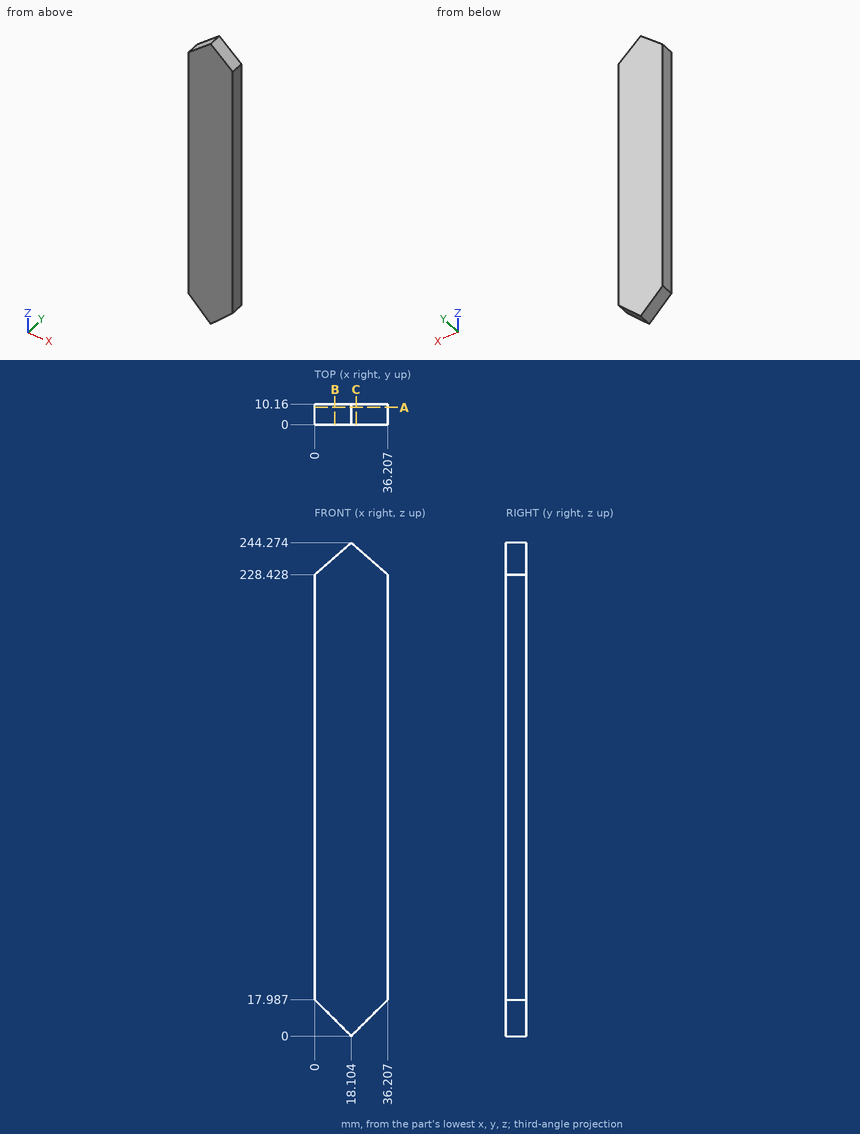
Geometry: see drawing. Coordinates: mm, zero at the bounding-box minimum. Coordinates: 2 decimals unless noted, no trailing zeros. Order: outer loops, then holes, each group sorted by start corner. A loop starts at its lowest first (then second) coordinate and runs counter-clockwise, first axis right, second up. Notation, with made-up numbers: (-18.5, 89.5) -> (-0.5, 89.5) arc R25 ccw to (-0.5, 109.5) -> close; hole circle Ø4 at (-39.75, 67.25). An arc over 180 degrees is marked (long way). Write each question's results on one line, items separated by ' | '. Start each with the question number.
1) Cut plane B-B, the plane x = 10. Output: boundary loops of the cut face in (y, z).
2) Material intervals for line 1 along Z through (x, y) = (14.5, 9); line 2 along Z through (x, y) = (13.5, 4.75) (1 decimal); line 3 along X through (y, z) = (7.5, 231), sorted ascending.
3) First-contact query: pin 1 (4 mm diameter, centred on x = 9.5, y = 7, fed in from +Z) (1 decimal); pin 2 (1.5 mm diameter, centred on x = 7, y = 2.5, fed in from +Z); pin 3 (4 mm diameter, centred on x = 22, y = 6.5, fed in from +Z) (1 decimal). Flat tips, straight axial feed; report the tip coordinate or a pass-through.
4) Cut plane A-A, the plane y = 8.5. Output: boundary loops of the cut face in (x, z), and give its area (3 significant figures).
5) Cut plane C-C, the plane x = 20.5. Output: boundary loops of the cut face in (y, z).
Checks:
1) outline: (0, 8.05) -> (10.16, 8.05) -> (10.16, 237.18) -> (0, 237.18) -> close
2) line 1: 3.58 to 241.12 | line 2: 4.6 to 240.2 | line 3: 2.94 to 33.27
3) pin 1: z = 238.5 | pin 2: z = 235.21 | pin 3: z = 242.6
4) outline: (0, 17.99) -> (18.1, 0) -> (36.21, 17.99) -> (36.21, 228.43) -> (18.1, 244.27) -> (0, 228.43) -> close | area: 8,230 mm^2
5) outline: (0, 2.38) -> (10.16, 2.38) -> (10.16, 242.18) -> (0, 242.18) -> close
